from build123d import *

# Parameters (mm, degrees)
BOSS_EXTRUDE1_DEPTH = 20
FILLET1_R           = 4
SKETCH3_R           = 6
CUT_EXTRUDE2_DEPTH  = 92.651513899


with BuildPart() as part:
    # Sketch2 → Boss-Extrude1 (new body)
    with BuildSketch(Plane.XY):
        with BuildLine():
            Line((-36, 0), (-40, 0))
            Line((-40, 0), (-40, -36))
            Line((-40, -36), (-24, -36))
            Line((-24, -36), (-24, -24))
            Line((-24, -24), (-30, -24))
            Line((-30, -24), (-30, 0))
            Line((-30, 0), (-24, 0))
            ThreePointArc((-24, 0), (0, 24), (24, 0))
            Line((24, 0), (30, 0))
            Line((30, 0), (30, -24))
            Line((30, -24), (24, -24))
            Line((24, -24), (24, -36))
            Line((24, -36), (40, -36))
            Line((40, -36), (40, 0))
            Line((40, 0), (36, 0))
            ThreePointArc((36, 0), (29.393876913, 20.784609691), (12, 33.941125497))
            Line((12, 33.941125497), (12, 44))
            Line((12, 44), (-12, 44))
            Line((-12, 44), (-12, 33.941125497))
            ThreePointArc((-12, 33.941125497), (-29.393876913, 20.784609691), (-36, 0))
        make_face()
    extrude(amount=-BOSS_EXTRUDE1_DEPTH)

    # Fillet1
    fillet1_edges = [part.edges().sort_by_distance(p)[0] for p in [
        (-36, 0, -10),
        (36, 0, -10),
    ]]
    fillet(fillet1_edges, radius=FILLET1_R)

    # Sketch3 → Cut-Extrude2 (cut, through all)
    with BuildSketch(Plane(origin=(0, 44, 0), x_dir=(1, 0, 0), z_dir=(0, 1, 0))):
        with Locations(Location((0, 10, 0), (0, 0, 270))):
            Circle(SKETCH3_R)
    extrude(amount=-CUT_EXTRUDE2_DEPTH, mode=Mode.SUBTRACT)


solid = part.part
Input: part model. Units: mm. Frame: model coordinates. A direction names the side the tool comes from. Coordinates: 2 decimals unless noted, no trailing zeros. Order: outer loops, then holes, each group sorted by start corner. A loop starts at its lowest first (then second) coordinate and runs counter-clockwise, first axis right, second up. Notation, with made-up numbers: M 61,74.5 L 74,74.5 A26 cw 74,90.5 Z; hole C 22.25,83 d8. An arc over 180 degrees is marked long. Write item = value, one per line. Start each with the question number.
(1) Section C-C on z = -6.25. Output: boundary loops of the cut face in (x, y), and give its area (3 significant figures).
(2) Line query: line 1 along Z through (x, y) = (0, 27); line 2 along X through (y, z) = (-18.5, -18.75); line 3 along X through (y, z) = (35.75, -10). Output: solid intervals per line, ascending. Write a range as [from, to].
(3) Reachability of faces 1 (the flat face through (-30, -12, -10)), 2 (the flat face through (12, 39, -10)), 3 (the cylindrical face through (1.802, 33.757, -4.277)), 4 (the flat face through (-24, -30, -10)) from +Z, -Z, +X, -X, +Y, -Y: full face, straight path, thin tool, end or side. Return the list, or none.
(4) Section B-B on x = 0. Output: boundary loops of the cut face in (y, z).
(5) Pull-direction query (Y, two-part tool) for faces 5 (the flat face through (-3, 25, -20)), 6 (the flat face through (32, -36, -10)), 7 (the flat face through (-27, 0, -10)); classes: released by +Y, released by -Y, zero draft, split by the parting line, or undercut.
(6) First-contact query: P1, Ø11, axis at x = 0, z = -10, coming from the +Y side; P2, Ø8, axis at x = -28, z = -13.5, coming from the +Y side; P3, Ø1.8, axis at x = 26, z = -7.5, coming from the +Y side; P4, Ø1.5, axis at x = -27.5, z = -7.5, coming from the +Y side. Flat tips, straight axial feed; report the tip coordinate or a pass-through.
(7) Section A-A on y = -17.5. Output: boundary loops of the cut face in (x, z).
(8) Section D-D on z = -2. Output: boundary loops of the cut face in (x, y), and give its area (3 significant figures).
Result set:
q1.outline = M -40,-36 L -24,-36 L -24,-24 L -30,-24 L -30,0 L -24,0 A24 cw -4.68,23.54 L -4.68,44 L -12,44 L -12,33.94 A36 ccw -35.82,3.6 A4 cw -39.8,0 L -40,0 Z; M 4.68,23.54 A24 cw 24,0 L 30,0 L 30,-24 L 24,-24 L 24,-36 L 40,-36 L 40,0 L 39.8,0 A4 cw 35.82,3.6 A36 ccw 12,33.94 L 12,44 L 4.68,44 Z
q1.area = 2,020 mm²
q2.line_1 = [-20, -16], [-4, 0]
q2.line_2 = [-40, -30], [30, 40]
q2.line_3 = [-12, -6], [6, 12]
q3.face_1 = +Z, -Z
q3.face_2 = +Z, -Z, +X, +Y
q3.face_3 = +Y, -Y
q3.face_4 = +Z, -Z, -Y
q4.outline = M 24,-20 L 44,-20 L 44,-16 L 24,-16 Z; M 24,-4 L 44,-4 L 44,0 L 24,0 Z
q5.face_5 = zero draft
q5.face_6 = released by -Y
q5.face_7 = undercut
q6.P1 = through
q6.P2 = 26.83
q6.P3 = 25.81
q6.P4 = 24.09
q7.outline = M -40,-20 L -30,-20 L -30,0 L -40,0 Z; M 30,-20 L 40,-20 L 40,0 L 30,0 Z
q8.outline = M -40,-36 L -24,-36 L -24,-24 L -30,-24 L -30,0 L -24,0 A24 cw 24,0 L 30,0 L 30,-24 L 24,-24 L 24,-36 L 40,-36 L 40,0 L 39.8,0 A4 cw 35.82,3.6 A36 ccw 12,33.94 L 12,44 L -12,44 L -12,33.94 A36 ccw -35.82,3.6 A4 cw -39.8,0 L -40,0 Z
q8.area = 2,210 mm²
